Input: part model. Units: mm. Frame: model coordinates. Coordinates: 2 decimals unless noted, no trailing zeros. Loops run counter-clockwise (first coordinate to the right, second up) from the corner with the lowest first, then second, coordinate; pieces in that order, holes last. Notation, with made-up numbers: (31.5, 46) - (57.5, 46) arc R26 cw to (57.5, 69) - close; hole circle Ø3 at (-1, -20). An arc over 180 degrees is marked (long way). Use one line per item in the form item = value.
Autodesk Inventor part; units mm, degrees
ref_plane "YZ Plane" through (0, 0, 0) normal (1, 0, 0) x (0, 1, 0)
ref_plane "XZ Plane" through (0, 0, 0) normal (0, 1, 0) x (-1, 0, 0)
ref_plane "XY Plane" through (0, 0, 0) normal (0, 0, 1) x (1, 0, 0)
sketch "Sketch1" plane through (0, 0, 0) normal (0, 0, 1) x (1, 0, 0)
  line L0 (2.8868, 0) -> (1.4434, -2.5)
  line L1 (1.4434, -2.5) -> (-1.4434, -2.5)
  line L2 (-1.4434, -2.5) -> (-2.8868, 0)
  line L3 (-2.8868, 0) -> (-1.4434, 2.5)
  line L4 (-1.4434, 2.5) -> (1.4434, 2.5)
  line L5 (1.4434, 2.5) -> (2.8868, 0)
  point P0 (0, 0)
  point P1 (0, 0)
  dimension "d0" = 5
extrude "Extrusion1" add sketch "Sketch1" along normal blind 7
sketch "Sketch2" plane through (0, 0, 7) normal (0, 0, 1) x (1, 0, 0)
  circle A0 centre (0, 0) radius 1.5
  dimension "d3" = 3
extrude "Extrusion2" add sketch "Sketch2" along normal blind 8
sketch "Sketch3" plane through (0, 0, 0) normal (0, 0, -1) x (-1, 0, 0)
  circle A0 centre (0, 0) radius 1.5
  dimension "d6" = 3
extrude "Extrusion3" cut sketch "Sketch3" against normal blind 4
sketch "Sketch4" plane through (0, 0, 4) normal (0, 0, -1) x (-1, 0, 0)
  circle A0 centre (0, 0) radius 1.5
extrude "Extrusion4" cut sketch "Sketch4" against normal through all
properties part number "Spacer7mm_m3_970070321"
Q1. Ray query, line 1 along Y through (x, z) = (0, 4.5); line 2 along X through (y, z) = (1.25, 3.5); line 3 along X through (y, z) = (-0.85, 6.25). Return the intervals inside material, ascending. Write a range as [from, to].
Check values:
line_1 = [-2.5, -1.5], [1.5, 2.5]
line_2 = [-2.17, -0.83], [0.83, 2.17]
line_3 = [-2.4, -1.24], [1.24, 2.4]
Q2. Pull-direction query (X, two-part tool) for faces 1 (the flat face through (1.24, 1.15, 7)), 2 (the flat face through (2.155, 1.267, 3.451)), 3 (the flat face through (-2.155, -1.267, 3.451)), 4 (the cylindrical face through (1.5, 0.07, 3.45)); classes: pulls with the +X half, pulls with the -X half, needs draft (parallel to the pull), parting line crosses it, or undercut.
Check values:
face_1 = needs draft
face_2 = pulls with the +X half
face_3 = pulls with the -X half
face_4 = undercut
Q3. Cut plane A-A, the plane x = 0. Return loops of the section in (y, z), then the cut area to 3 significant figures.
Check values:
outline = (-2.5, 0) - (-1.5, 0) - (-1.5, 7) - (-2.5, 7) - close; (1.5, 0) - (2.5, 0) - (2.5, 7) - (1.5, 7) - close
area = 14.0 mm²
Q4. Cut plane D-D, the plane y = -1.8. Return loops of the section in (x, z).
Check values:
outline = (-1.85, 0) - (1.85, 0) - (1.85, 7) - (-1.85, 7) - close
Q5. Cut plane B-B, the plane y = 0.3. Return loops of the section in (x, z), then the cut area to 3 significant figures.
Check values:
outline = (-2.71, 0) - (-1.47, 0) - (-1.47, 7) - (-2.71, 7) - close; (1.47, 0) - (2.71, 0) - (2.71, 7) - (1.47, 7) - close
area = 17.4 mm²
Q6. Cut plane C-C, the plane z = 5. Return loops of the section in (x, y).
Check values:
outline = (-2.89, 0) - (-1.44, -2.5) - (1.44, -2.5) - (2.89, 0) - (1.44, 2.5) - (-1.44, 2.5) - close; hole circle Ø3 at (0, 0)
